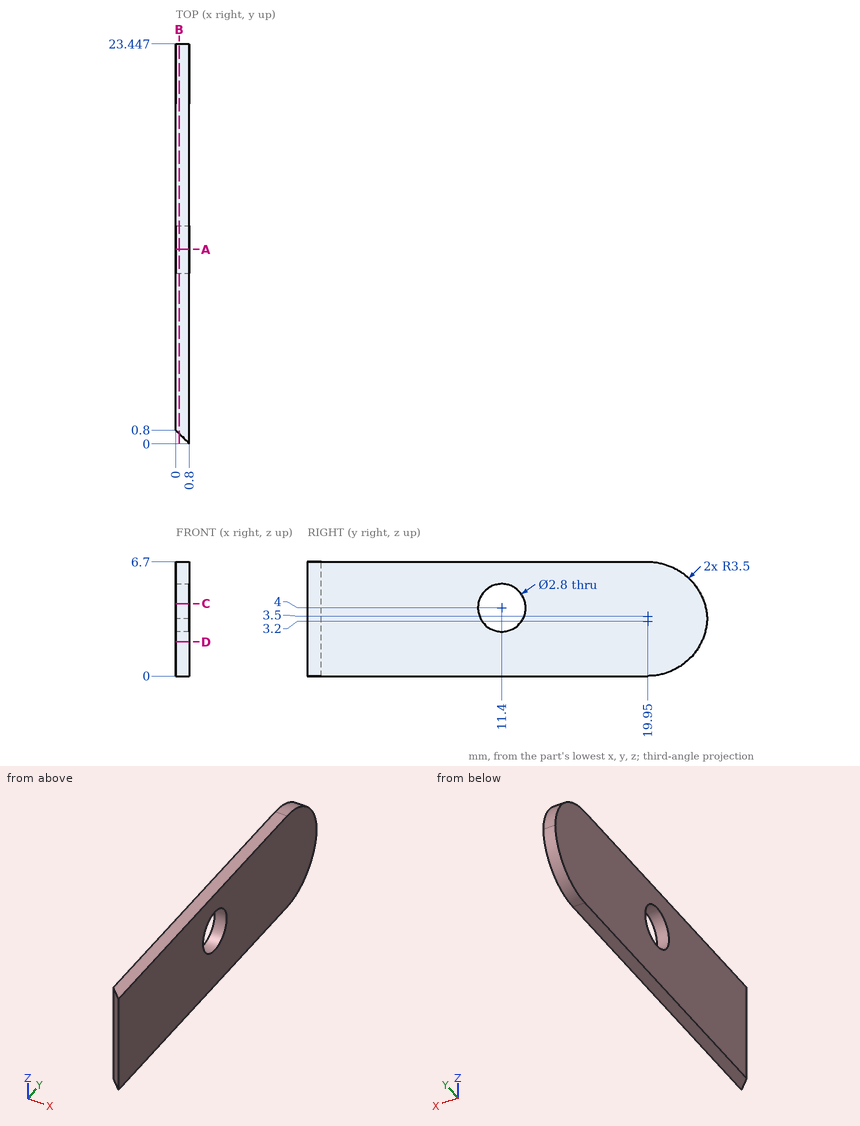
Geometry check sheet. Reference: drawing and pictorial views, mm from the part's lowest x, y, z. Round coordinates to 2 decimals unless told otherwise and drop trailing zeros. Order: outer loops, then holes, each group sorted by start corner. A loop starts at its lowest first (then second) coordinate and runs counter-clockwise, first axis right, second up. Notation, with made-up numbers: M 48,26 L 98,26 A7 ccw 98,37 Z; hole C -20,37 d5. An arc over 180 degrees is marked long. One line per item, written item: value. Start each with the question number.
1. Section check A-A on y = 11.4. Enter the section's corners in (x, z), and give its area (3 significant figures).
2. Section check C-C on z = 4.25. Enter the section's corners in (x, y), and give its area (3 significant figures).
3. Section check D-D on z = 2. Enter the section's corners in (x, y).
4. Section check B-B on x = 0.2. Enter the section's corners in (y, z), and give its area (3 significant figures).
5. Gauge pin test, flat end, axial feed: P1, Ø2, axis at y = 11.5, z = 4, coming from the +X side. Record the tip position at first contact, or that the pin passes through.
6. Scan lines: line 1 along Y through (x, z) = (0.35, 4); line 2 along Y through (x, z) = (0.6, 4); line 3 along Y through (x, z) = (0.15, 1). Record each from-to range of solid material in increasing order.
Results found:
1. outline: M 0,0 L 0.8,0 L 0.8,2.6 L 0,2.6 Z; M 0,5.4 L 0.8,5.4 L 0.8,6.7 L 0,6.7 Z
1. area: 3.12 mm^2
2. outline: M 0,0.8 L 0.8,0 L 0.8,10.02 L 0,10.02 Z; M 0,12.78 L 0.8,12.78 L 0.8,23.29 L 0,23.29 Z
2. area: 16.1 mm^2
3. outline: M 0,0.8 L 0.8,0 L 0.8,23.11 L 0,23.11 Z
4. outline: M 0.6,0 L 19.95,0 A3.5 ccw 23.45,3.35 A3.5 ccw 19.95,6.7 L 0.6,6.7 Z; hole C 11.4,4 d2.8
4. area: 142 mm^2
5. P1: through
6. line 1: 0.45 to 10, 12.8 to 23.36
6. line 2: 0.2 to 10, 12.8 to 23.36
6. line 3: 0.65 to 22.4
